```python
from build123d import *

# Parameters (mm, degrees)
F1_DEPTH = 101.6
F2_W     = 19.05
F2_H     = 12.7
F3_DEPTH = 152.4
F4_R     = 6.35
F5_DEPTH = 50.8
F6_W     = 152.4
F6_H     = 15.875
F7_DEPTH = 50.8
F9_DEPTH = 15.875
F10_R    = 12.7


with BuildPart() as f1:
    # F0 (on Front) → F1 (new body)
    with BuildSketch(Plane.XZ):
        Polygon((76.2, 25.4), (-76.2, 25.4), (-76.2, -25.4), (-38.1, -25.4), (-38.1, -12.7), (38.1, -12.7), (38.1, -25.4), (76.2, -25.4), align=None)
    extrude(amount=-F1_DEPTH)

    # F2 (on face) → F3 (cut)
    with BuildSketch(Plane.YZ.offset(76.2)):
        Polygon((53.975, 12.7), (38.1, 12.7), (38.1, 0), (88.9, 0), (88.9, 12.7), (73.025, 12.7), align=None)
        with Locations((63.5, 19.05)):
            Rectangle(F2_W, F2_H)
    extrude(amount=-F3_DEPTH, mode=Mode.SUBTRACT)

    # F4 (on face) → F5 (cut, through all)
    with BuildSketch(Plane.XY.offset(25.4)):
        with Locations((57.15, 19.05)):
            Circle(F4_R)
        with Locations((-57.15, 19.05)):
            Circle(F4_R)
    extrude(amount=-F5_DEPTH, mode=Mode.SUBTRACT)

    # F6 (on face) → F7 (join, symmetric)
    with BuildSketch(Plane.XY.offset(25.4)):
        with Locations((0, 109.5375)):
            Rectangle(F6_W, F6_H)
    extrude(amount=F7_DEPTH, both=True)

    # F8 (on face) → F9 (cut, through all)
    with BuildSketch(Plane.XZ.offset(-101.6)):
        with BuildLine():
            Line((38.1, 76.2), (-38.1, 76.2))
            ThreePointArc((-38.1, 76.2), (0, 38.1), (38.1, 76.2))
        make_face()
    extrude(amount=-F9_DEPTH, mode=Mode.SUBTRACT)

    # F10
    f10_edges = [f1.edges().sort_by_distance(p)[0] for p in [
        (-76.2, 109.5375, 76.2),
        (76.2, 109.5375, 76.2),
    ]]
    fillet(f10_edges, radius=F10_R)


solid = f1.part
```
Model file for the job. Use its own axes, mm. A direction names the side the tool comes from. Coordinates: 2 decimals unless noted, no trailing zeros. Loops run counter-clockwise (first coordinate to the right, second up) from the corner with the lowest first, then second, coordinate; pieces in that order, holes last. Notation, with made-up numbers: (67.5, 9.25) - (98.5, 9.25) arc R23 cw to (98.5, 20.25) - close; hole circle Ø2 at (69.5, 79). An arc over 180 degrees is marked (long way). Write item = value, one per line. Start each with the question number.
Item 1: Wall check: probe 1 along X at (y, z) = (19, -14); probe 2 along X at (y, z) = (19, -10); probe 3 along Y at (x, z) = (-57.15, 5) (3 decimals). Give the ranges that are in metal, low to high. Write a range as [from, to].
Item 2: Saw through at A-A, the plane z = 6. List the corners of the cut face in (x, y) (3 decimals).
Item 3: Pull direction Y, two halves, no side cores. Call faces 1 (the face through (-1, 0, 0)), 2 (the face through (1, 63, 0)), 3 (the face through (-51, 110, 76.2)): +Y half, -Y half, draft (parallel to the pull), parting line (faces both ways), or undercut.
Item 4: 3-axis set-ups, long thin cutter, end or side, ignore diameter. For faces 4 (the face through (-1, 117.475, 15)), 5 (the face through (-38.1, 50, -19)), 6 (the face through (72.38, 109.65, 72.58)), 7 (the face through (1, 87, 25.4)), 8 (the face through (1, 81, 12.7)): which of +Z, -Z, +X, -X, +Y, -Y reach the whole face in a straight line?
Item 5: Saw through at D-D, the plane x = 45. List the corners of the cut face in (y, z) (3 decimals), then the cut area to 3 significant figures.
Item 6: Drop flat-ended pins along their axis: pin 1 Ø23 at (x, y) = (6, 92.5) entering from +Z; pin 2 Ø7.5 at (x, y) = (-57.15, 19.05) entering from +Z; pin 3 Ø10 at (x, y) = (-33.5, 25) entering from +Z; pin 4 Ø5 at (x, y) = (-19.5, 47) entering from -Z. Give the stop position or say it passes through.
Item 7: Saw through at C-C, the plane x = -57.15. List the corners of the cut face in (y, z) (3 decimals), then the cut area to 3 significant figures.
Item 8: Saw through at B-B, the plane y = 19.05. List the corners of the cut face in (x, z).
Answers:
q1.probe_1 = [-76.2, -63.5], [-50.8, -38.1], [38.1, 50.8], [63.5, 76.2]
q1.probe_2 = [-76.2, -63.5], [-50.8, 50.8], [63.5, 76.2]
q1.probe_3 = [0, 12.7], [25.4, 38.1], [88.9, 117.475]
q2.outline = (-76.2, 0) - (76.2, 0) - (76.2, 38.1) - (-76.2, 38.1) - close; (-76.2, 88.9) - (76.2, 88.9) - (76.2, 117.475) - (-76.2, 117.475) - close; hole circle Ø12.7 at (-57.15, 19.05); hole circle Ø12.7 at (57.15, 19.05)
q3.face_1 = -Y half
q3.face_2 = undercut
q3.face_3 = draft
q4.face_4 = +Z, -Z, +X, -X, +Y
q4.face_5 = -Z, -Y
q4.face_6 = +Z, +X, +Y, -Y
q4.face_7 = +Z, +X, -X, -Y
q4.face_8 = +X, -X
q5.outline = (0, -25.4) - (117.475, -25.4) - (117.475, 76.2) - (101.6, 76.2) - (101.6, 25.4) - (73.025, 25.4) - (73.025, 12.7) - (88.9, 12.7) - (88.9, 0) - (38.1, 0) - (38.1, 12.7) - (53.975, 12.7) - (53.975, 25.4) - (0, 25.4) - close
q5.area = 5,890 mm2
q6.pin_1 = 40.4
q6.pin_2 = through
q6.pin_3 = 25.4
q6.pin_4 = -12.7
q7.outline = (0, -25.4) - (12.7, -25.4) - (12.7, 25.4) - (0, 25.4) - close; (25.4, -25.4) - (117.475, -25.4) - (117.475, 76.2) - (101.6, 76.2) - (101.6, 25.4) - (73.025, 25.4) - (73.025, 12.7) - (88.9, 12.7) - (88.9, 0) - (38.1, 0) - (38.1, 12.7) - (53.975, 12.7) - (53.975, 25.4) - (25.4, 25.4) - close
q7.area = 5,240 mm2
q8.outline = (-76.2, -25.4) - (-63.5, -25.4) - (-63.5, 25.4) - (-76.2, 25.4) - close; (-50.8, -25.4) - (-38.1, -25.4) - (-38.1, -12.7) - (38.1, -12.7) - (38.1, -25.4) - (50.8, -25.4) - (50.8, 25.4) - (-50.8, 25.4) - close; (63.5, -25.4) - (76.2, -25.4) - (76.2, 25.4) - (63.5, 25.4) - close
